Can you work these out from the model? Positions are in its coordinate system, mm. A direction names the side the tool comes from. Round coordinates to 2 decimals unless told otherwise and drop trailing zeros. Order: outer loops, then holes, each group sorted by start corner. A loop starts at its lowest first (then second) coordinate and runs counter-clockwise, first axis right, second up. Notation, with made-up numbers: (10.25, -10) - (62.25, -10) arc R30 cw to (62.25, 13) - close; hole circle Ø5 at (68, 51.25). An arc over 180 degrees is marked (long way). Write item = value, one per line.
Autodesk Fusion 360 part; units mm, degrees
sketch "Sketch1" plane through (0, 0, 0) normal (0, 0, 1) x (1, 0, 0) in component "Figet Spinner"
  circle A0 centre (0, 0) radius 25 construction
  line L0 (0, 0) -> (0, 37) construction
  line L1 (-3.7528, 31.5) -> (-7.5056, 25)
  line L2 (-7.5056, 25) -> (-3.7528, 18.5)
  line L3 (-3.7528, 18.5) -> (3.7528, 18.5)
  line L4 (3.7528, 18.5) -> (7.5056, 25)
  line L5 (7.5056, 25) -> (3.7528, 31.5)
  line L6 (3.7528, 31.5) -> (-3.7528, 31.5)
  spline S0 degree 5 poles (-7.5138, 31.9717) (-7.2318, 32.4496) (-6.6528, 33.3792) (-5.7393, 34.6951) (-4.4298, 36.2901) (-2.6362, 38.0009) (-0.6893, 39.4059) (1.3878, 40.4856) (3.5405, 41.2348) (5.6614, 41.6834) (7.5834, 41.9073) (8.8194, 41.9749) (9.5098, 41.9954) (9.8557, 42) (10, 42) knots 0 0 0 0 0 0 0.1 0.2 0.3 0.4 0.5 0.6 0.7 0.8 0.9 1 1 1 1 1 1
  line L7 (9, 42) -> (11, 42)
  spline S1 degree 5 poles (10, 42) (9.5694, 41.4679) (8.784, 40.4086) (7.8329, 38.8347) (7.0266, 36.7666) (6.8325, 34.2352) (7.3693, 32.2479) (8.175, 30.7821) (8.8868, 29.8139) (9.2884, 29.3289) (9.2944, 29.3216) knots 0 0 0 0 0 0 0.1 0.2 0.3 0.4 0.5 0.501529 0.501529 0.501529 0.501529 0.501529 0.501529
  line L8 (8.3624, 30.4454) -> (10.2264, 28.1979)
  circle A1 centre (0, 0) radius 11
  spline S2 degree 5 poles (-23.9314, -22.493) (-24.4863, -22.4877) (-25.5808, -22.451) (-27.1772, -22.3179) (-29.2133, -21.9813) (-31.5916, -21.2835) (-33.7818, -20.2999) (-35.7555, -19.0409) (-37.4806, -17.5512) (-38.9296, -15.9388) (-40.0844, -14.3862) (-40.7611, -13.3496) (-41.124, -12.762) (-41.3009, -12.4647) (-41.3731, -12.3397) knots 0 0 0 0 0 0 0.1 0.2 0.3 0.4 0.5 0.6 0.7 0.8 0.9 1 1 1 1 1 1
  spline S3 degree 5 poles (-41.3731, -12.3397) (-40.6969, -12.4466) (-39.3869, -12.5972) (-37.5483, -12.6339) (-35.3541, -12.2981) (-33.0648, -11.2004) (-31.6122, -9.742) (-30.7456, -8.3113) (-30.263, -7.2107) (-30.0438, -6.6205) (-30.0405, -6.6116) knots 0 0 0 0 0 0 0.1 0.2 0.3 0.4 0.5 0.501529 0.501529 0.501529 0.501529 0.501529 0.501529
  line L9 (-25.4034, -6) -> (-29.1562, -12.5)
  line L10 (-29.1562, -12.5) -> (-25.4034, -19)
  line L11 (-25.4034, -19) -> (-17.8979, -19)
  line L12 (-17.8979, -19) -> (-14.1451, -12.5)
  line L13 (-14.1451, -12.5) -> (-17.8979, -6)
  line L14 (-17.8979, -6) -> (-25.4034, -6)
  spline S4 degree 5 poles (31.4452, -9.4787) (31.7181, -9.9619) (32.2336, -10.9281) (32.9164, -12.3772) (33.643, -14.3087) (34.2278, -16.7174) (34.4712, -19.106) (34.3677, -21.4447) (33.9401, -23.6836) (33.2682, -25.7446) (32.5011, -27.521) (31.9416, -28.6253) (31.6142, -29.2335) (31.4452, -29.5353) (31.3731, -29.6603) knots 0 0 0 0 0 0 0.1 0.2 0.3 0.4 0.5 0.6 0.7 0.8 0.9 1 1 1 1 1 1
  spline S5 degree 5 poles (31.3731, -29.6603) (31.1275, -29.0213) (30.6029, -27.8115) (29.7154, -26.2009) (28.3275, -24.4685) (26.2323, -23.0347) (24.2429, -22.506) (22.5706, -22.4708) (21.3762, -22.6032) (20.7554, -22.7084) (20.7461, -22.71) knots 0 0 0 0 0 0 0.1 0.2 0.3 0.4 0.5 0.501529 0.501529 0.501529 0.501529 0.501529 0.501529
  line L15 (17.8979, -19) -> (25.4034, -19)
  line L16 (25.4034, -19) -> (29.1562, -12.5)
  line L17 (29.1562, -12.5) -> (25.4034, -6)
  line L18 (25.4034, -6) -> (17.8979, -6)
  line L19 (17.8979, -6) -> (14.1451, -12.5)
  line L20 (14.1451, -12.5) -> (17.8979, -19)
  arc A2 (-8.464, 19.2188) -> (-20.8759, -2.2793) centre (0, 0) ccw
  arc A3 (-12.4119, -16.9394) -> (12.4119, -16.9394) centre (0, 0) ccw
  arc A4 (20.8759, -2.2793) -> (8.464, 19.2188) centre (0, 0) ccw
  arc A5 (-18.5686, -22.2757) -> (18.5686, -22.2757) centre (0, 0) ccw
  arc A6 (28.5756, -4.9431) -> (10.007, 27.2188) centre (0, 0) ccw
  arc A7 (-8.464, 19.2188) -> (8.464, 19.2188) centre (0, 25) ccw
  arc A8 (-7.5138, 31.9717) -> (-10.007, 27.2187) centre (0, 25) ccw
  arc A9 (18.5686, -22.2757) -> (20.7461, -22.71) centre (21.6506, -12.5) ccw
  arc A10 (31.4452, -9.4787) -> (28.5756, -4.9431) centre (21.6506, -12.5) ccw
  arc A11 (20.8759, -2.2793) -> (12.4119, -16.9394) centre (21.6506, -12.5) ccw
  arc A12 (-10.007, 27.2187) -> (-28.5756, -4.9431) centre (0, 0) ccw
  arc A13 (-28.5756, -4.9431) -> (-30.0405, -6.6116) centre (-21.6506, -12.5) ccw
  arc A14 (-23.9314, -22.493) -> (-18.5686, -22.2757) centre (-21.6506, -12.5) ccw
  arc A15 (-12.4119, -16.9394) -> (-20.8759, -2.2793) centre (-21.6506, -12.5) ccw
  arc A16 (10.007, 27.2187) -> (9.2944, 29.3217) centre (0, 25) ccw
  arc A17 (7.7553, 31.702) -> (7.7553, 31.702) centre (0, 25) ccw
  point P0 (0, 25)
  point P1 (3, 41)
  point P2 (-37.007, -17.9019)
  point P3 (-31.3324, -9.1347)
  point P4 (34.007, -23.0981)
  point P5 (23.5771, -22.5673)
  dimension "d14" = 50
  dimension "d15" = 6.5
  dimension "d16" = 31.5
  dimension "d17" = 20.5
  dimension "d18" = 22
extrude "Extrude2" add sketch "Sketch1" along normal mid plane 8 contours S1 A7 A8 A16 A17 | S0 S1 A17 | S2 S3 S4 S5 A2 A3 A4 A5 A6 A9 A10 A11 A12 A13 A14 A15 A17 in component "Figet Spinner"
extrude "Extrude3" add sketch "Sketch1" along normal mid plane 7 contours A2 A3 A4 A7 A11 A15 A17 in component "Figet Spinner"
component "Figet Spinner" placed x (1, 0, 0) y (0, 1, 0) z (0, 0, 1) at (0, 0, 0)
(1) Will these pins go through, and if not, where does the flat tip stop? P1, Ø4, axis at y = 32, z = -1, coming from the -X side; P2, Ø3, axis at x = -24, z = 2, coming from the -Y side; P3, Ø2.5, axis at x = -22.5, z = 1, coming from the +Y side.
Computed:
P1 = -8.95
P2 = -22.71
P3 = 19.73
(2) On a 3-axis mill with a long thin cutter (end or side, diameter ignored), from which of +Z, -Z, +X, -X, +Y, -Y can I reach the whole of each face in a straight line? I mean faces 1 (the face through (-18.3, 10.3, 3.7)), 2 (the face through (-5.66, 21.8, -0.06)), 3 (the face through (9.703, 28.304, -0.056)). Say none if no direction works.
Computed:
face_1 = +Z
face_2 = +Z, -Z
face_3 = +Z, -Z, +X
(3) If we section it at A-A (y = 0): Write out the boundary of the cut face in (x, z).
Computed:
outline = (-29, -4) - (-21, -4) - (-21, -3.5) - (-11, -3.5) - (-11, 3.5) - (-21, 3.5) - (-21, 4) - (-29, 4) - close; (11, -3.5) - (21, -3.5) - (21, -4) - (29, -4) - (29, 4) - (21, 4) - (21, 3.5) - (11, 3.5) - close
(4) If we section it at B-B (x = -20): Write out the boundary of the cut face in (y, z).
Computed:
outline = (-22.62, -4) - (-19, -4) - (-19, 4) - (-22.62, 4) - close; (-6, -4) - (-2.38, -4) - (-2.38, -3.5) - (6.4, -3.5) - (6.4, -4) - (21, -4) - (21, 4) - (6.4, 4) - (6.4, 3.5) - (-2.38, 3.5) - (-2.38, 4) - (-6, 4) - close
(5) If we section it at C-C (z = -2.5): State how many separate pieces and enclosed holes the cut face has, plus the area to 3 significant figures.
Computed:
separate_pieces = 1
enclosed_holes = 4
area = 2,320 mm^2
(6) If I drill on line 1 (X direction, y = -0.5, z = 0.5); line 2 (Y direction, x = 0, z = 0); line 3 (Y direction, x = 9, z = 0.5), over which ranges is the centre line in solid material (lowest first)? Write a range as from..to.
Computed:
line_1 = -29..-10.99, 10.99..29
line_2 = -29..-11, 11..18.5, 31.5..39.71
line_3 = -27.57..-6.32, 6.32..29.69, 40.65..41.97
(7) Thinking about a two-plate mould opening in Y: for faces 4 (the face through (13.23, -6.93, 4)), 5 (the face through (-21.2, -22.74, -0.06)), 6 (the face through (0.2, -21, 3.7)), which applies, +Y half, -Y half, draft (parallel to the pull), parting line (faces both ways), or undercut?
Computed:
face_4 = draft
face_5 = -Y half
face_6 = undercut
